from build123d import *

# Parameters (mm, degrees)
F1_DEPTH     = 16.2
F3_DEPTH     = 10
F4_T4_DEPTH  = 5
F4_T10_DEPTH = 5


# Not quite as in the source:
# - a fillet or chamfer that OpenCascade refuses, or shapes differently, is made with other operations: its cross-section is extruded or revolved along the edge and cut away or added


with BuildPart() as f1:
    # F0 (on Front) → F1 (new body)
    with BuildSketch(Plane.XZ):
        Polygon((-29.15, 0), (0, 0), (29.15, 0), (29.15, -18.5), (34.15, -18.5), (34.15, 5), (0, 5), (-34.15, 5), (-34.15, -18.5), (-29.15, -18.5), align=None)
    extrude(amount=F1_DEPTH)

    # F2 (on face) → F3 (join)
    with BuildSketch(Plane.XZ.offset(16.2)):
        Polygon((34.15, 5), (-34.15, 5), (-34.15, 0), (-29.15, 0), (29.15, 0), (34.15, 0), align=None)
    extrude(amount=F3_DEPTH)

    # F4: chamfer of 10 x 19 on 2 edges, made by hand


with BuildPart() as f4_tool2:
    # F4_s3 → F4_t4 (new body)
    with BuildSketch(Plane.YZ.offset(29.15)):
        Polygon((-26.2, 0), (-16.2, -19), (-16.2, 0), align=None)
    extrude(amount=F4_T4_DEPTH)

    split(bisect_by=Plane.XZ.offset(26.2), keep=Keep.BOTTOM)

    split(bisect_by=Plane.XY.offset(-18.5), keep=Keep.TOP)


with BuildPart() as f1_1:
    add(f1.part)

    # F4_t1: union F4_tool2
    add(f4_tool2.part)


with BuildPart() as f4_tool8:
    # F4_s9 → F4_t10 (new body)
    with BuildSketch(Plane.YZ.offset(-34.15)):
        Polygon((-26.2, 0), (-16.2, -19), (-16.2, 0), align=None)
    extrude(amount=F4_T10_DEPTH)

    split(bisect_by=Plane.XZ.offset(26.2), keep=Keep.BOTTOM)

    split(bisect_by=Plane.XY.offset(-18.5), keep=Keep.TOP)


with BuildPart() as f1_2:
    add(f1_1.part)

    # F4_t7: union F4_tool8
    add(f4_tool8.part)


solid = f1_2.part
CAD build for the part. Positions are in the model's coordinates, mm. A direction names the side the tool comes from. Round coordinates to 2 decimals unless told otherwise and drop trailing zeros. Write each loop counter-clockwise with the first axis right and the second up, starting at its lowest first coordinate (ties: lowest second). Pieces come first, ordered by that corner, then holes. Notation, with made-up numbers: M -16,53 L 10,53 A13 ccw 10,61 Z; hole C -20.75,89 d3. An arc over 180 degrees is marked long. Use a Markdown table: item, result. Add a question column.
1. Drill centre lines: probe 1 along X at (y, z) = (-19, -10.25); probe 2 along Z at (x, y) = (-10, -16.25); probe 3 along Y at (x, z) = (30.5, -16.75). Where is each one in solid material? Low to high.
2. Slice it at C-C on x = 18. Give the cut face in (y, z).
3. 3-axis set-ups, long thin cutter, end or side, ignore diameter. For faces 1 (the face through (0, 0, 1)), 2 (the face through (-29.15, -10, -9)): which of +Z, -Z, +X, -X, +Y, -Y reach the whole face in a straight line?
4. Flat gauge pin, fed straight in: P1, Ø3, axis at x = 20, y = -3, coming from the -Z side. Where does the tip first touch, or does it go through?
5. Slice it at A-A on z = -4. Give the cut face in (x, y), then the cut area to 3 significant figures.
6. Slice it at D-D on z = -11. Give the cut face in (x, y), then the cut area to 3 significant figures.
7. Slice it at B-B on y = -19.5. Give the cut face in (x, z), then the cut area to 3 significant figures.
Reply:
| question | item | result |
|---|---|---|
| 1 | probe 1 | x = -34.15 to -29.15, 29.15 to 34.15 |
| 1 | probe 2 | z = 0 to 5 |
| 1 | probe 3 | y = -17.38 to 0 |
| 2 | outline | M -26.2,0 L 0,0 L 0,5 L -26.2,5 Z |
| 3 | face 1 | +Z, -Z, +X, -X, +Y |
| 3 | face 2 | -Z, +Y, -Y |
| 4 | P1 | stops at z = 0 |
| 5 | outline | M -34.15,-24.09 L -29.15,-24.09 L -29.15,0 L -34.15,0 Z; M 29.15,-24.09 L 34.15,-24.09 L 34.15,0 L 29.15,0 Z |
| 5 | area | 241 mm^2 |
| 6 | outline | M -34.15,-20.41 L -29.15,-20.41 L -29.15,0 L -34.15,0 Z; M 29.15,-20.41 L 34.15,-20.41 L 34.15,0 L 29.15,0 Z |
| 6 | area | 204 mm^2 |
| 7 | outline | M -34.15,-12.73 L -29.15,-12.73 L -29.15,0 L 29.15,0 L 29.15,-12.73 L 34.15,-12.73 L 34.15,5 L -34.15,5 Z |
| 7 | area | 469 mm^2 |
